The model under review builds one solid part; all positions refer to its coordinate system, in mm. Face numbers are marked on the shaded views. Give positions to 0.01 mm unless a question says otherwise; leave off trailing zeros. Order: outer loops, then holes, each group sorted by start corner. A loop starts at its lowest first (then second) coordinate and runs counter-clockwise, first axis right, second up. Notation, with made-up numbers: (14.25, 33.5) - (64.25, 33.5) arc R13 ccw to (64.25, 47.5) - close; hole circle Ø7 at (34, 19). An arc over 180 degrees is marked (long way). Use CSV: the item, a comma, the result in double quotes. Start each with the question number.
1. Take a section at A-A, the plane x = 51. State the section outline as (y, z) points.
2. Take a section at B-B, the plane z = 12. State the section outline as (x, y) points.
3. For pin 1 (12 mm diameter, centred on y = 13, z = 13.5, fed in from -X); pin 2 (12 mm diameter, centred on x = 24, y = 11.5, fed in from +Z); pin 3 (8 mm diameter, centred on y = -12.5, z = 10.5, fed in from +X), all flat-tipped, find the tip position at first contact; note any pin that passes through.
4. Draft analysis for pull direction Z (two halves, no side actions). For the marked faces 1, 2, 3 and 4, state which applies: released by +Z, released by -Z, zero draft, split by the parting line, or undercut.
5. To check wall thickness, follow line 1 (Y direction, x = 0, z = 22); line 2 (Z direction, x = -51.5, y = 5.5); line 3 (Y direction, x = -90, z = 2.6). State the ranges of each line that lie inside material, in increasing order. Write a range as [from, to].
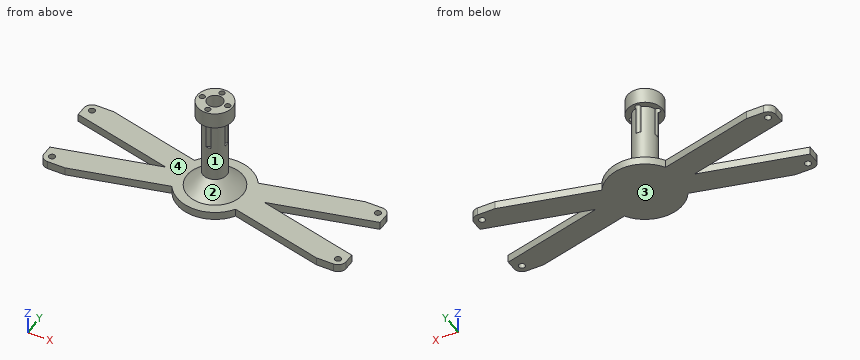
```python
from build123d import *

# Parameters (mm, degrees)
ESBO_O1_R                = 23.75
RESSALTO_EXTRUS_O1_DEPTH = 5
ESBO_O8_R                = 2
RESSALTO_EXTRUS_O2_DEPTH = 5
ESBO_O9_R                = 7.5
ESBO_O9_R_2              = 5
RESSALTO_EXTRUS_O3_DEPTH = 60
RESSALTO_EXTRUS_O4_START = -10
ESBO_O10_R               = 11
ESBO_O10_R_2             = 5
RESSALTO_EXTRUS_O4_DEPTH = 10
ESBO_O11_R               = 1.75
CORTE_EXTRUS_O1_DEPTH    = 28
PADR_OCIRCULAR2_COUNT    = 4
CHANFRO1_SIZE            = 10
FILETE1_R                = 5
FILETE1_OF_ESPELHAR4_R   = 5
ESPELHAR5_OUTLINE_R      = 2
ESPELHAR5_DEPTH          = 5


# Read off the part's stored shape, not the designer's step: Espelhar5
with BuildPart() as part:
    # Esboço1 → Ressalto-extrusão1 (new body)
    with BuildSketch(Plane.XY):
        Circle(ESBO_O1_R)
    extrude(amount=RESSALTO_EXTRUS_O1_DEPTH)

    # Esboço8 → Ressalto-extrusão2 (add)
    with BuildSketch(Plane.XY.offset(5)):
        Polygon((-20.042848617, 12.741535202), (-79.076707808, 27.5), (-95, 27.5), (-95, 16.019176952), (-23.680882993, -1.8106023), align=None)
        with Locations((-90, 22.5)):
            Circle(ESBO_O8_R, mode=Mode.SUBTRACT)
    ressalto_extrus_o2 = extrude(amount=-RESSALTO_EXTRUS_O2_DEPTH)

    # Esboço9 → Ressalto-extrusão3 (add)
    with BuildSketch(Plane.XY.offset(5)):
        Circle(ESBO_O9_R)
        Circle(ESBO_O9_R_2, mode=Mode.SUBTRACT)
    extrude(amount=RESSALTO_EXTRUS_O3_DEPTH)

    # Esboço10 → Ressalto-extrusão4 (add)
    with BuildSketch(Plane.XY.offset(65).offset(RESSALTO_EXTRUS_O4_START)):
        Circle(ESBO_O10_R)
        Circle(ESBO_O10_R_2, mode=Mode.SUBTRACT)
    extrude(amount=RESSALTO_EXTRUS_O4_DEPTH)

    # Esboço11 → Corte-extrusão1 (cut)
    with BuildSketch(Plane.XY.offset(65)):
        with Locations((0, -8)):
            Circle(ESBO_O11_R)
    corte_extrus_o1 = extrude(amount=-CORTE_EXTRUS_O1_DEPTH, mode=Mode.SUBTRACT)

    # PadrãoCircular2: Corte-extrusão1 ×4 about axis
    padr_ocircular2_axis = Axis((0, 0, 0), (0, 0, 1))
    for i in range(1, PADR_OCIRCULAR2_COUNT):
        add(corte_extrus_o1.rotate(padr_ocircular2_axis, i * 360 / PADR_OCIRCULAR2_COUNT), mode=Mode.SUBTRACT)

    # Chanfro1
    chanfro1_edges = [part.edges().sort_by_distance(p)[0] for p in [
        (-7.5, 0, 5),
    ]]
    chamfer(chanfro1_edges, length=CHANFRO1_SIZE)

    # Filete1
    filete1_edges = [part.edges().sort_by_distance(p)[0] for p in [
        (-95, 27.5, 2.5),
    ]]
    fillet(filete1_edges, radius=FILETE1_R)

    # Espelhar4: Ressalto-extrusão2 across plane
    add(ressalto_extrus_o2.mirror(Plane.ZX))

    # Filete1 of Espelhar4
    filete1_of_espelhar4_edges = [part.edges().sort_by_distance(p)[0] for p in [
        (-95, -27.5, 2.5),
    ]]
    fillet(filete1_of_espelhar4_edges, radius=FILETE1_OF_ESPELHAR4_R)

    # Espelhar5 outline → Espelhar5 (add)
    with BuildSketch(Plane.XY):
        with BuildLine():
            Line((95, -22.5), (95, -16.019176952))
            Line((95, -16.019176952), (30.923292192, 0))
            Line((30.923292192, 0), (95, 16.019176952))
            Line((95, 16.019176952), (95, 22.5))
            ThreePointArc((95, 22.5), (93.535533906, 26.035533906), (90, 27.5))
            Line((90, 27.5), (79.076707808, 27.5))
            Line((79.076707808, 27.5), (20.042848617, 12.741535202))
            ThreePointArc((20.042848617, 12.741535202), (23.75, 0), (20.042848617, -12.741535202))
            Line((20.042848617, -12.741535202), (79.076707808, -27.5))
            Line((79.076707808, -27.5), (90, -27.5))
            ThreePointArc((90, -27.5), (93.535533906, -26.035533906), (95, -22.5))
        make_face()
        with Locations((90, -22.5)):
            Circle(ESPELHAR5_OUTLINE_R, mode=Mode.SUBTRACT)
        with Locations((90, 22.5)):
            Circle(ESPELHAR5_OUTLINE_R, mode=Mode.SUBTRACT)
    extrude(amount=ESPELHAR5_DEPTH)


solid = part.part
```
Determined:
1,outline,"(-20.48, 0) - (-5.02, 0) - (-5.02, 5) - (-20.48, 5) - close; (5.02, 0) - (20.48, 0) - (20.48, 5) - (5.02, 5) - close"
2,outline,"circle Ø21 at (0, 0); hole circle Ø10 at (0, 0)"
3,pin 1,"stops at x = -10.11"
3,pin 2,"stops at z = 5"
3,pin 3,"stops at x = 11.37"
4,face 1,"undercut"
4,face 2,"undercut"
4,face 3,"released by -Z"
4,face 4,"released by +Z"
5,line 1,"y = [-7.5, -5], [5, 7.5]"
5,line 2,"z = [0, 5]"
5,line 3,"y = [-27.5, -24.5], [-20.5, -14.77], [14.77, 20.5], [24.5, 27.5]"
